Design review of the part built by this model. Coordinates are the model's own, in mm. A direction names the side the tool comes from. Give positions to 0.01 mm unless a question says otherwise; leave off trailing zeros. Loops run counter-clockwise (first coordinate to the right, second up) from the corner with the lowest first, then second, coordinate; pieces in that order, holes last. Notation, with made-up numbers: (82, 66.25) -> (89, 66.25) arc R16 ccw to (89, 73.25) -> close; hole circle Ø6 at (25, -21.75). An arc over 180 degrees is marked (long way). Use a Markdown table: item, result. Add a question column.
1. Add section A-A (z = 95). State the section outline as (x, y) points (3 decimals), and give its area (3 significant figures).
2. To check wall thickness, follow line 1 (Z direction, x = 0, y = -1.4) (3 decimals); line 2 (X direction, y = 0.95, z = -53.5); line 3 (Z direction, x = 1.5, y = -1.45). State the ranges of each line that lie inside material, in increasing order.
3. Draft analysis for pull direction Z (two halves, no side actions). For faces 6 (the flat face through (0, -2.5, -1)), 7 (the flat face through (5, 0, -55)), 8 (the cylindrical face through (-13, 0, 104)), state which applies: pulls with the +Z half, pulls with the -Z half, needs draft (parallel to the pull), parting line crosses it, or undercut.
4. For faces 1 (the flat face through (7.5, 0, -108)), 2 (the flat face through (0, 0, 105)), 3 (the flat face through (-11, 0, -105)), 4 (the flat face through (-5, 0, -55)), 5 (the flat face through (0, 0, -110)), list the 3-axis set-ups (+Z, -Z, +X, -X, +Y, -Y) from which the entire face can be reached by the end or side of a thin tool; tool diameter is ignored.
5. Add section D-D (x = 13). State the section outline as (y, z) points.
6. Add section B-B (y = 1.65). State the section outline as (x, z) points (3 decimals), and give its area (3 significant figures).
7. Add section C-C (x = 0). State the section outline as (y, z) points (3 decimals), and give its area (3 significant figures).
8. For pin 1 Ø6 at (x, z) = (0, 95) entering from -Y; pin 2 Ø1.5 at (y, z) = (0.5, -108.5) entering from -X, all flat-tipped, find the tip position at first contact; note any pin that passes through.
```python
from build123d import *

# Parameters (mm, degrees)
F0_W     = 15
F0_H     = 5
F1_DEPTH = 2.5
F3_D     = 5.25
F4_R     = 5
F5_W     = 10
F5_H     = 50
F6_DEPTH = 10


with BuildPart() as f1:
    # F0 (on Front) → F1 (new body, symmetric)
    with BuildSketch(Plane.XZ):
        Polygon((15, -105), (15, 105), (-15, 105), (-15, -105), (-7.5, -105), (-7.5, -100), (7.5, -100), (7.5, -105), align=None)
        with Locations((0, -107.5)):
            Rectangle(F0_W, F0_H)
        with Locations((0, -102.5)):
            Rectangle(F0_W, F0_H)
    extrude(amount=F1_DEPTH, both=True)

    # F3 (through all)
    with Locations(Plane.XZ.offset(2.5)):
        with Locations((0, 95)):
            Hole(F3_D / 2)

    # F4
    f4_edges = [f1.edges().sort_by_distance(p)[0] for p in [
        (15, 0, 105),
        (-15, 0, 105),
    ]]
    fillet(f4_edges, radius=F4_R)

    # F5 (on face) → F6 (cut)
    with BuildSketch(Plane.XZ.offset(2.5)):
        with Locations((0, -55)):
            Rectangle(F5_W, F5_H)
    extrude(amount=-F6_DEPTH, mode=Mode.SUBTRACT)


solid = f1.part
```
Taken from the geometry:
| question | item | result |
|---|---|---|
| 1 | outline | (-15, -2.5) -> (-2.625, -2.5) -> (-2.625, 2.5) -> (-15, 2.5) -> close; (2.625, -2.5) -> (15, -2.5) -> (15, 2.5) -> (2.625, 2.5) -> close |
| 1 | area | 124 mm^2 |
| 2 | line 1 | z = -110 to -80, -30 to 92.375, 97.625 to 105 |
| 2 | line 2 | x = -15 to -5, 5 to 15 |
| 2 | line 3 | z = -110 to -80, -30 to 92.85, 97.15 to 105 |
| 3 | face 6 | needs draft |
| 3 | face 7 | undercut |
| 3 | face 8 | pulls with the +Z half |
| 4 | face 1 | -Z, +X, +Y, -Y |
| 4 | face 2 | +Z, +X, -X, +Y, -Y |
| 4 | face 3 | -Z, -X, +Y, -Y |
| 4 | face 4 | +Y, -Y |
| 4 | face 5 | -Z, +X, -X, +Y, -Y |
| 5 | outline | (-2.5, -105) -> (2.5, -105) -> (2.5, 104) -> (-2.5, 104) -> close |
| 6 | outline | (-15, -105) -> (-7.5, -105) -> (-7.5, -110) -> (7.5, -110) -> (7.5, -105) -> (15, -105) -> (15, 100) arc R5 ccw to (10, 105) -> (-10, 105) arc R5 ccw to (-15, 100) -> close; hole (-5, -80) -> (5, -80) -> (5, -30) -> (-5, -30) -> close; hole circle Ø5.25 at (0, 95) |
| 6 | area | 5,840 mm^2 |
| 7 | outline | (-2.5, -110) -> (2.5, -110) -> (2.5, -80) -> (-2.5, -80) -> close; (-2.5, -30) -> (2.5, -30) -> (2.5, 92.375) -> (-2.5, 92.375) -> close; (-2.5, 97.625) -> (2.5, 97.625) -> (2.5, 105) -> (-2.5, 105) -> close |
| 7 | area | 799 mm^2 |
| 8 | pin 1 | stops at y = -2.5 |
| 8 | pin 2 | stops at x = -7.5 |
